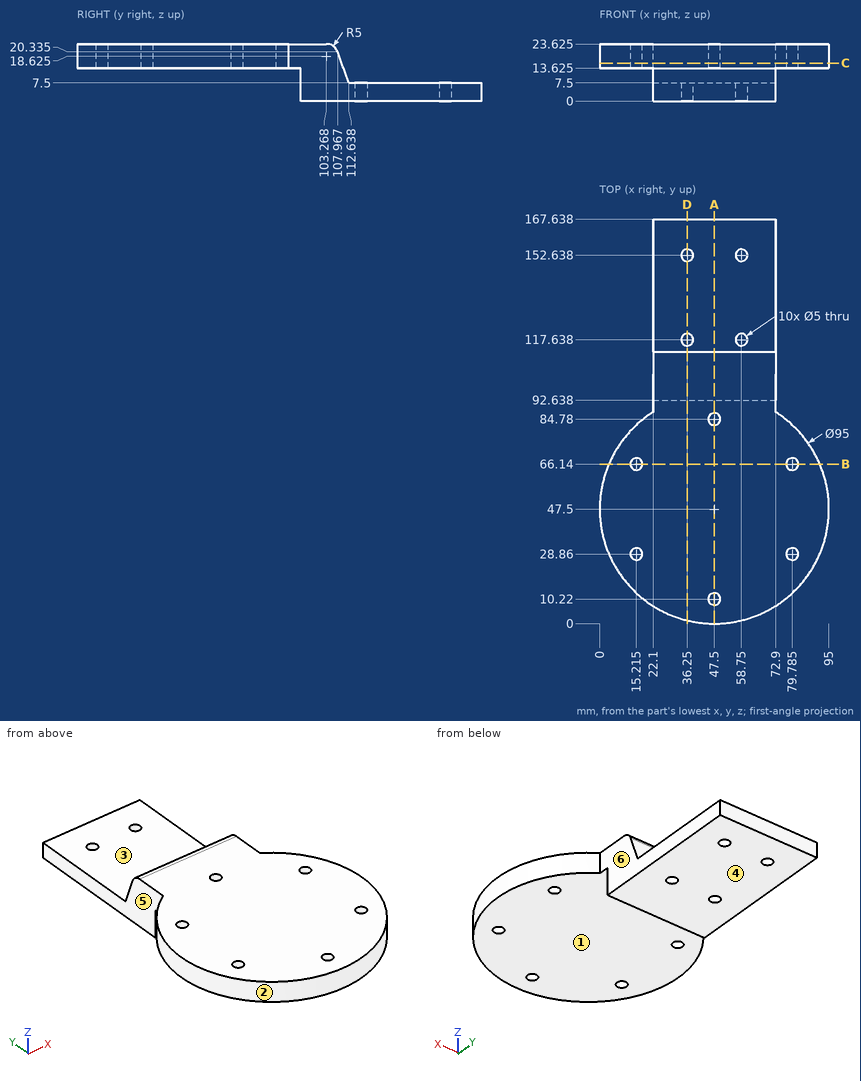
Answer from the drawing. Dimensions are ordinates in mm from the lowest x, y and z of the part. A direction names the side the tool comes from. Coordinates: 2 decimals unless noted, no trailing zeros. Write each loop counter-clockwise with the first axis right and the second up, starting at its lowest first coordinate (ties: lowest second). Pieces come first, ordered by that corner, then holes. Notation, with made-up numbers: (12, -17) - (25, -17) arc R17 ccw to (25, -13) - close; hole circle Ø10 at (-9.5, -26). An arc over 180 degrees is marked (long way). Answer as CSV lines item,"result".
1. Straight lines are drawn through the part: line 1 (Y direction, x = 36.25, z = 6); line 2 (Z direction, x = 37, y = 41.5) (1 decimal); line 3 (Y direction, x = 14, z = 15.5) (1 decimal). For each, find the intervals that lie inside material, in ascending order. Write a range as [from, to].
Computed values:
line 1,"y = [92.64, 115.14], [120.14, 150.14], [155.14, 167.64]"
line 2,"z = [13.6, 23.6]"
line 3,"y = [13.8, 26.7], [31, 64], [68.3, 81.2]"
2. Find section A-A (x = 47.5). Give the vertices of the cut face in (y, z) (1 decimal), plus the area to 3 significant figures.
Computed values:
outline,"(0, 13.6) - (7.7, 13.6) - (7.7, 23.6) - (0, 23.6) - close; (12.7, 13.6) - (82.3, 13.6) - (82.3, 23.6) - (12.7, 23.6) - close; (87.3, 13.6) - (92.6, 13.6) - (92.6, 0) - (167.6, 0) - (167.6, 7.5) - (112.6, 7.5) - (108, 20.3) arc R5 ccw to (103.3, 23.6) - (87.3, 23.6) - close"
area,"1,660 mm²"
3. Find section B-B (y = 66.14). Give the vertices of the cut face in (x, z) (1 decimal).
Computed values:
outline,"(3.8, 13.6) - (12.7, 13.6) - (12.7, 23.6) - (3.8, 23.6) - close; (17.7, 13.6) - (77.3, 13.6) - (77.3, 23.6) - (17.7, 23.6) - close; (82.3, 13.6) - (91.2, 13.6) - (91.2, 23.6) - (82.3, 23.6) - close"
4. Find section C-C (z = 15.75). Give the vertices of the cut face in (x, y) (1 decimal).
Computed values:
outline,"(22.1, 87.6) arc R47.5 ccw (long way) to (72.9, 87.6) - (72.9, 109.6) - (22.1, 109.6) - close; hole circle Ø5 at (15.2, 28.9); hole circle Ø5 at (15.2, 66.1); hole circle Ø5 at (47.5, 10.2); hole circle Ø5 at (47.5, 84.8); hole circle Ø5 at (79.8, 28.9); hole circle Ø5 at (79.8, 66.1)"
5. Determine the mould class of the marked faces 4, 5 and 6 for opening direction X: +X half, -X half, draft (parallel to the pull), parting line (faces both ways), or undercut.
Computed values:
face 4,"draft"
face 5,"-X half"
face 6,"+X half"
6. Find section D-D (x = 36.25). Give the vertices of the cut face in (y, z) (1 decimal).
Computed values:
outline,"(1.4, 13.6) - (92.6, 13.6) - (92.6, 0) - (115.1, 0) - (115.1, 7.5) - (112.6, 7.5) - (108, 20.3) arc R5 ccw to (103.3, 23.6) - (1.4, 23.6) - close; (120.1, 0) - (150.1, 0) - (150.1, 7.5) - (120.1, 7.5) - close; (155.1, 0) - (167.6, 0) - (167.6, 7.5) - (155.1, 7.5) - close"
7. A tool of negligible diameter and unlimited length cuts with its end or side. For the marked faces 1, 2 and 3, from which of +Z, -Z, +X, -X, +Y, -Y can it reach the whole face along a straight path? Write none if from no direction.
Computed values:
face 1,"-Z, +X, -X, -Y"
face 2,"+Z, -Z"
face 3,"+Z, +X, -X, +Y"
8. Given P1, Ø10, axis at x = 42.5, z = 3.5, coming from the -Y side; P2, Ø8, axis at x = 79.79, y = 28.86, coming from the -Z side (3 decimals); P3, Ø10, axis at y = 133.5, z = 4.5, coming from the +X side, each flat-ended and moving along its own axis, determine where each tip first touches the part or whether it passes through.
Computed values:
P1,"stops at y = 92.64"
P2,"stops at z = 13.625"
P3,"stops at x = 72.9"
